```python
from build123d import *
from build123d.topology import SkipClean

# Parameters (mm, degrees)
SKETCH1_W                     = 10
SKETCH1_H                     = 170.55
SKETCH1_R                     = 2.5
BOSS_EXTRUDE1_DEPTH           = 2
SKETCH2_W                     = 10
SKETCH2_H                     = 170.55
SKETCH2_R                     = 2.95
BOSS_EXTRUDE2_DEPTH           = 1
SKETCH3_W                     = 69.85
SKETCH3_H                     = 10.16
SKETCH3_R                     = 1.86055
BOSS_EXTRUDE3_DEPTH           = 2.5
FILLET1_START                 = -1
FILLET1_DEPTH                 = 10.16
FILLET1_START_2               = -17.7000001
FILLET1_2_DEPTH               = 35.4000001
FILLET1_START_3               = -5
FILLET1_3_DEPTH               = 10
SKETCH4_W                     = 10
SKETCH4_H                     = 13.05
BOSS_EXTRUDE4_DEPTH           = 3
SKETCH4_3_W                   = 3.175
SKETCH4_3_H                   = 38.1
BOSS_EXTRUDE5_DEPTH           = 11.1125
SKETCH5_W                     = 7.38125
SKETCH5_H                     = 38.1
BOSS_EXTRUDE6_DEPTH           = 50.8
SKETCH6_W                     = 3.690625
SKETCH6_H                     = 38.1
CUT_EXTRUDE1_DEPTH            = 44.45
CHAMFER1_SIZE                 = 4.7625
CHAMFER1_SIZE_2               = 8.248891971
SKETCH7_W                     = 69.85
SKETCH7_H                     = 10.16
CUT_EXTRUDE2_DEPTH            = 145.5
SKETCH8_W                     = 31.75
SKETCH8_H                     = 38.1
BOSS_EXTRUDE7_DEPTH           = 3.175
SKETCH9_W                     = 10
SKETCH9_H                     = 3.175
SKETCH9_W_2                   = 16.35
SKETCH9_H_2                   = 3
CUT_EXTRUDE3_DEPTH            = 74.579605063
CHAMFER2_SIZE                 = 6.35
CHAMFER3_SIZE                 = 6.35
SKETCH11_W                    = 1.7
SKETCH11_H                    = 58.9125
M3_CLEARANCE_HOLE1_AT_2_COUNT = 2
M3_CLEARANCE_HOLE1_AT_2_PITCH = 25.4
SKETCH13_W                    = 10
SKETCH13_H                    = 6.35
BOSS_EXTRUDE8_DEPTH           = 3.175


with BuildPart() as part:
    # Sketch1 → Boss-Extrude1 (new body)
    with BuildSketch(Plane.XY):
        with Locations((0, 3)):
            Rectangle(SKETCH1_W, SKETCH1_H)
        with Locations((0, 82.275)):
            Circle(SKETCH1_R, mode=Mode.SUBTRACT)
    extrude(amount=BOSS_EXTRUDE1_DEPTH)

    # Sketch2 → Boss-Extrude2 (add)
    with BuildSketch(Plane(origin=(0, 0, 0), x_dir=(-1, 0, 0), z_dir=(0, 0, -1))):
        with Locations((0, 3)):
            Rectangle(SKETCH2_W, SKETCH2_H)
        with Locations((0, 82.275)):
            Circle(SKETCH2_R, mode=Mode.SUBTRACT)
    extrude(amount=BOSS_EXTRUDE2_DEPTH)

    # Sketch3 → Boss-Extrude3 (add)
    with BuildSketch(Plane.XZ.offset(82.275)):
        with Locations((0, 4.08)):
            Rectangle(SKETCH3_W, SKETCH3_H)
        with Locations(Location((28.575, 4.08, 0), (0, 0, 270))):
            Circle(SKETCH3_R, mode=Mode.SUBTRACT)
        with Locations(Location((-28.575, 4.08, 0), (0, 0, 270))):
            Circle(SKETCH3_R, mode=Mode.SUBTRACT)
    extrude(amount=-BOSS_EXTRUDE3_DEPTH)

    # Fillet1: read off the stored shape, not the designer's step
    # Fillet1 outline → Fillet1 (add)
    with BuildSketch(Plane.XY.offset(FILLET1_START)):
        with BuildLine():
            Line((5, -79.775), (17.7, -79.775))
            ThreePointArc((17.7, -79.775), (8.719743879, -76.055256121), (5, -67.075))
            Line((5, -67.075), (5, -79.775))
        make_face()
        with BuildLine():
            Line((-17.7, -79.775), (-5, -79.775))
            Line((-5, -79.775), (-5, -67.075))
            ThreePointArc((-5, -67.075), (-8.719743879, -76.055256121), (-17.7, -79.775))
        make_face()
    extrude(amount=FILLET1_DEPTH)

    # Fillet1 2 outline → Fillet1 2 (cut)
    with BuildSketch(Plane.YZ.offset(FILLET1_START_2)):
        with BuildLine():
            Line((-66, 9.16), (-79.775009155, 9.160018885))
            ThreePointArc((-79.775009155, 9.160018885), (-75.089891257, 3.937849653), (-68.347034302, 2))
            Line((-68.347034302, 2), (-66, 2))
            Line((-66, 2), (-66, 9.16))
        make_face()
    extrude(amount=FILLET1_2_DEPTH, mode=Mode.SUBTRACT)

    # Fillet1 3 outline → Fillet1 3 (add)
    with BuildSketch(Plane.YZ.offset(FILLET1_START_3)):
        with BuildLine():
            ThreePointArc((-68.347034302, 2), (-75.089891257, 3.937849653), (-79.775009155, 9.160018885))
            Line((-79.775009155, 9.160018885), (-79.775, 0))
            Line((-79.775, 0), (-66, 0))
            Line((-66, 0), (-66, 2))
            Line((-66, 2), (-68.347034302, 2))
        make_face()
    extrude(amount=FILLET1_3_DEPTH)

    # Sketch4 → Boss-Extrude4 (add)
    with SkipClean():  # the faces are left unmerged after this step: merging them gives an invalid solid
        with BuildSketch(Plane(origin=(0, 0, -1), x_dir=(-1, 0, 0), z_dir=(0, 0, -1))):
            Polygon((8.175, 63.225), (8.175, 101.325), (5, 101.325), (5, 88.275), (5, 63.225), align=None)
            with Locations((0, 94.8)):
                Rectangle(SKETCH4_W, SKETCH4_H)
            Polygon((-5, 88.275), (-5, 101.325), (-8.175, 101.325), (-8.175, 63.225), (-5, 63.225), align=None)
        extrude(amount=-BOSS_EXTRUDE4_DEPTH)

    # Sketch4<3> → Boss-Extrude5 (add)
    with SkipClean():  # the faces are left unmerged after this step: merging them gives an invalid solid
        with BuildSketch(Plane(origin=(0, 0, -1), x_dir=(-1, 0, 0), z_dir=(0, 0, -1))):
            with Locations((6.5875, 82.275)):
                Rectangle(SKETCH4_3_W, SKETCH4_3_H)
            with Locations((-6.5875, 82.275)):
                Rectangle(SKETCH4_3_W, SKETCH4_3_H)
        extrude(amount=-BOSS_EXTRUDE5_DEPTH)

    # Sketch5 → Boss-Extrude6 (add)
    with SkipClean():  # the faces are left unmerged after this step: merging them gives an invalid solid
        with BuildSketch(Plane.XY.offset(10.1125)):
            with Locations((-4.484375, 82.275)):
                Rectangle(SKETCH5_W, SKETCH5_H)
            with Locations((4.484375, 82.275)):
                Rectangle(SKETCH5_W, SKETCH5_H)
        extrude(amount=BOSS_EXTRUDE6_DEPTH)

    # Sketch6 → Cut-Extrude1 (cut)
    with SkipClean():  # the faces are left unmerged after this step: merging them gives an invalid solid
        with BuildSketch(Plane.XY.offset(60.9125)):
            with Locations((-6.3296875, 82.275)):
                Rectangle(SKETCH6_W, SKETCH6_H)
            with Locations((6.3296875, 82.275)):
                Rectangle(SKETCH6_W, SKETCH6_H)
        extrude(amount=-CUT_EXTRUDE1_DEPTH, mode=Mode.SUBTRACT)

    # Chamfer1
    # the kernel refuses this chamfer: 8.248891971, 4.7625 mm, written as the material it takes off along each edge
    with BuildSketch(Plane(origin=(-0.79375, 122.66559091, 10.1125), x_dir=(-1, 0, 0), z_dir=(0, -1, 0))) as chamfer1_piece_1_section:
        Polygon((CHAMFER1_SIZE, 0), (0, -CHAMFER1_SIZE_2), (0, 0), align=None)
    chamfer1_piece_1 = extrude(amount=80.78118182, mode=Mode.PRIVATE)
    chamfer1_piece_1 = split(chamfer1_piece_1, bisect_by=Plane(origin=(-5, 122.66559091, 10.1125), z_dir=(1, 0, 0)), keep=Keep.TOP, mode=Mode.PRIVATE)
    add(chamfer1_piece_1, mode=Mode.SUBTRACT)
    with BuildSketch(Plane(origin=(0.79375, 122.66559091, 10.1125), x_dir=(1, 0, 0), z_dir=(0, -1, 0))) as chamfer1_piece_2_section:
        Polygon((CHAMFER1_SIZE, 0), (0, CHAMFER1_SIZE_2), (0, 0), align=None)
    chamfer1_piece_2 = extrude(amount=80.78118182, mode=Mode.PRIVATE)
    chamfer1_piece_2 = split(chamfer1_piece_2, bisect_by=Plane(origin=(5, 122.66559091, 10.1125), z_dir=(-1, 0, 0)), keep=Keep.TOP, mode=Mode.PRIVATE)
    add(chamfer1_piece_2, mode=Mode.SUBTRACT)

    # Sketch7 → Cut-Extrude2 (cut)
    with BuildSketch(Plane.XZ.offset(82.275)):
        with Locations((0, 4.08)):
            Rectangle(SKETCH7_W, SKETCH7_H)
    extrude(amount=-CUT_EXTRUDE2_DEPTH, mode=Mode.SUBTRACT)


with BuildPart() as cut_extrude2_kept_piece:
    # of the separate pieces the step leaves, the one the design keeps (cut_extrude2_pieces_kept)
    add(part.part.solids().sort_by_distance((-8.175, 63.225, -1))[0])

    # Sketch8 → Boss-Extrude7 (add)
    with BuildSketch(Plane(origin=(0, 0, 2), x_dir=(-1, 0, 0), z_dir=(0, 0, -1))):
        with Locations((0, 82.275)):
            Rectangle(SKETCH8_W, SKETCH8_H)
    extrude(amount=-BOSS_EXTRUDE7_DEPTH)

    # Sketch9 → Cut-Extrude3 (cut, through all)
    with BuildSketch(Plane(origin=(0, 101.325, 0), x_dir=(1, 0, 0), z_dir=(0, 1, 0))):
        with Locations((0, -3.5875)):
            Rectangle(SKETCH9_W, SKETCH9_H)
        with Locations((0, -0.5)):
            Rectangle(SKETCH9_W_2, SKETCH9_H_2)
    extrude(amount=-CUT_EXTRUDE3_DEPTH, mode=Mode.SUBTRACT)


with BuildPart() as cut_extrude3_piece_1:
    # of the separate pieces the step leaves, piece 1, a body of its own (cut_extrude3_pieces)
    add(cut_extrude2_kept_piece.part.solids().sort_by_distance((-15.875, 101.325, 2))[0])

    # Chamfer3
    # the kernel refuses this chamfer: 6.35 mm, written as the material it adds along each edge
    with BuildSketch(Plane(origin=(-4.484375, 101.325, 16.4625), x_dir=(-1, 0, 0), z_dir=(0, -1, 0))) as chamfer3_piece_1_section:
        Polygon((CHAMFER3_SIZE, 0), (0, -CHAMFER3_SIZE), (0, 0), align=None)
    chamfer3_piece_1 = extrude(amount=38.1, mode=Mode.PRIVATE)
    chamfer3_piece_1 = split(chamfer3_piece_1, bisect_by=Plane(origin=(-8.175, 101.325, 16.4625), z_dir=(1, 0, 0)), keep=Keep.TOP, mode=Mode.PRIVATE)
    add(chamfer3_piece_1)

    # Sketch11 → M3 Clearance Hole1 (revolve, cut)
    with BuildSketch(Plane(origin=(-12.7, 82.275, 2), x_dir=(0, 1, 0), z_dir=(1, 0, 0))):
        with Locations((0.85, 29.45625)):
            Rectangle(SKETCH11_W, SKETCH11_H)
    m3_clearance_hole1 = revolve(axis=Axis((-12.7, 82.275, -4.35), (0, 0, 1)), mode=Mode.SUBTRACT)



with BuildPart() as cut_extrude3_piece_2:
    # of the separate pieces the step leaves, piece 2, a body of its own (cut_extrude3_pieces)
    add(cut_extrude2_kept_piece.part.solids().sort_by_distance((15.875, 101.325, 2))[0])

    # Chamfer2
    # the kernel refuses this chamfer: 6.35 mm, written as the material it adds along each edge
    with BuildSketch(Plane(origin=(4.484375, 101.325, 16.4625), x_dir=(1, 0, 0), z_dir=(0, -1, 0))) as chamfer2_piece_1_section:
        Polygon((CHAMFER2_SIZE, 0), (0, CHAMFER2_SIZE), (0, 0), align=None)
    chamfer2_piece_1 = extrude(amount=38.1, mode=Mode.PRIVATE)
    chamfer2_piece_1 = split(chamfer2_piece_1, bisect_by=Plane(origin=(8.175, 101.325, 16.4625), z_dir=(-1, 0, 0)), keep=Keep.TOP, mode=Mode.PRIVATE)
    add(chamfer2_piece_1)

    # M3 Clearance Hole1 at 2: M3 Clearance Hole1 ×2
    with Locations(*[(i * M3_CLEARANCE_HOLE1_AT_2_PITCH, 0, 0) for i in range(1, M3_CLEARANCE_HOLE1_AT_2_COUNT)]):
        add(m3_clearance_hole1, mode=Mode.SUBTRACT)


with BuildPart() as cut_extrude3_piece_1_1:
    add(cut_extrude3_piece_1.part)

    add(cut_extrude3_piece_2.part)  # Boss-Extrude8 merges Cut-Extrude3 piece 2
    # Sketch13 → Boss-Extrude8 (add)
    with BuildSketch(Plane(origin=(0, 0, 2), x_dir=(-1, 0, 0), z_dir=(0, 0, -1))):
        with Locations((0, 98.15)):
            Rectangle(SKETCH13_W, SKETCH13_H)
        with Locations((0, 66.4)):
            Rectangle(SKETCH13_W, SKETCH13_H)
    extrude(amount=-BOSS_EXTRUDE8_DEPTH)


solid = cut_extrude3_piece_1_1.part
```
Here's how the part is built. I have some questions about the finished solid (model axes, mm). A direction names the side the tool comes from. Round coordinates to 2 decimals unless told otherwise and drop trailing zeros. Order: outer loops, then holes, each group sorted by start corner. A loop starts at its lowest first (then second) coordinate and runs counter-clockwise, first axis right, second up. Notation, with made-up numbers: M 39,84 L 62,84 A21 ccw 62,114 Z; hole C 36.5,-27.5 d9. An arc over 180 degrees is marked long. Answer in a Markdown table with one row per item.
Item 1: I'm going to push flat-ended pins straight in: pin 1 (2.5 mm diameter, centred on y = 84.5, z = 7.5, fed in from +X) (3 decimals); pin 2 (1 mm diameter, centred on x = 3, y = 92, fed in from -Z); pin 3 (1 mm diameter, centred on x = 11.5, y = 94.5, fed in from +Z) (3 decimals). Where does each tip first touch, or does it pass through?
A:
| item | result |
|---|---|
| pin 1 | stops at x = 8.175 |
| pin 2 | stops at z = 13.67 |
| pin 3 | stops at z = 5.175 |
Item 2: Imagine slicing it at A-A, the plane z = 34.5. Write out the boundary of the cut face in (x, y) (3 decimals).
A:
| item | result |
|---|---|
| outline | M -4.484,63.225 L -0.794,63.225 L -0.794,101.325 L -4.484,101.325 Z; M 0.794,63.225 L 4.484,63.225 L 4.484,101.325 L 0.794,101.325 Z |
Item 3: If I drill on L1, parallel to Y at x = -12.7, z = 2.65 (3 decimals); L2, parallel to X at y = 65, z = 42; L3, parallel to X at y = 70, z = 19 (3 decimals), over which ranges is the centre line in solid material (lowest first)? Write a range as from..to.
A:
| item | result |
|---|---|
| L1 | y = 63.225..80.575, 83.975..101.325 |
| L2 | x = -4.48..-0.79, 0.79..4.48 |
| L3 | x = -8.175..-0.794, 0.794..8.175 |
Item 4: For faces 1 (the face through (10, 83, 5.175)), 2 (the face through (0, 69.575, 4)), 3 (the face through (0.794, 82, 39)), 4 (the face through (2.926, 82.542, 14.668)), 5 (the face through (-4.484, 82, 42)), which set-ups out of +Z, -Z, +X, -X, +Y, -Y let a thin tool reach every point of the face, with its end or its side?
A:
| item | result |
|---|---|
| face 1 | +Z, +X, +Y, -Y |
| face 2 | -Z |
| face 3 | +Z, +Y, -Y |
| face 4 | +Y, -Y |
| face 5 | +Z, -X, +Y, -Y |
Item 5: Thinking about a two-plate mould opening in Z: for faces 6 (the face through (-2.926, 82.542, 14.668)), 7 (the face through (6.356, 82.542, 20.941)), 8 (the face through (0, 94.975, 4)), 9 (the face through (-7, 83, 2)), which applies, +Z half, -Z half, draft (parallel to the pull), parting line (faces both ways), or undercut?
A:
| item | result |
|---|---|
| face 6 | undercut |
| face 7 | +Z half |
| face 8 | draft |
| face 9 | -Z half |
Item 6: Imagine slicing it at C-C, the plane x = -12.7. Write out the boundary of the cut face in (y, z) (3 decimals).
A:
| item | result |
|---|---|
| outline | M 63.225,2 L 80.575,2 L 80.575,5.175 L 63.225,5.175 Z; M 83.975,2 L 101.325,2 L 101.325,5.175 L 83.975,5.175 Z |
Item 7: Imagine slicing it at B-B, the plane y = 93. Write out the boundary of the cut face in (x, z) (1 decimal).
A:
| item | result |
|---|---|
| outline | M -15.9,2 L -5,2 L -5,11.1 L -0.8,18.4 L -0.8,60.9 L -4.5,60.9 L -4.5,22.8 L -8.2,19.1 L -8.2,5.2 L -15.9,5.2 Z; M 0.8,18.4 L 5,11.1 L 5,2 L 15.9,2 L 15.9,5.2 L 8.2,5.2 L 8.2,19.1 L 4.5,22.8 L 4.5,60.9 L 0.8,60.9 Z |
